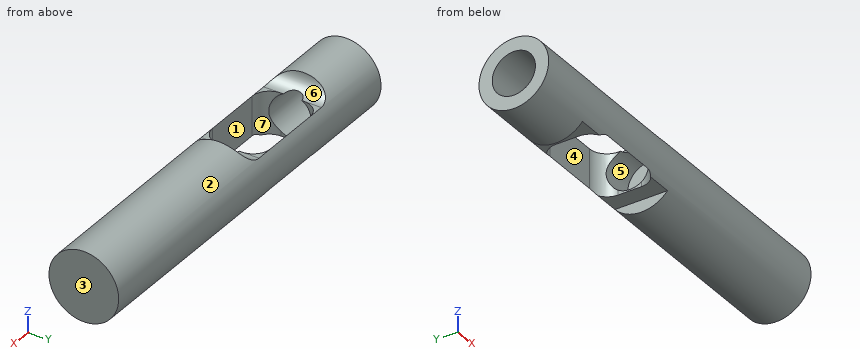
```python
from build123d import *

# Parameters (mm, degrees)
F0_W     = 115.125928
F0_H     = 10.15817
F2_W     = 37.343366
F2_H     = 12.383293
F3_DEPTH = 25
F4_R     = 6.295086
F5_DEPTH = 59.5
F7_DEPTH = 25


with BuildPart() as f1:
    # F0 (on Front) → F1 (revolve)
    with BuildSketch(Plane.XZ):
        with Locations((-1.547912, 5.079085)):
            Rectangle(F0_W, F0_H)
    revolve(axis=Axis((-1.547912, 0, 0), (-1, 0, 0)))

    # F2 (on Front) → F3 (cut, symmetric)
    with BuildSketch(Plane.XZ):
        with BuildLine():
            Line((-3.192568, 19.639129), (-40.535934, 19.639129))
            Line((-40.535934, 19.639129), (-40.535934, 10.707924))
            ThreePointArc((-40.535934, 10.707924), (-39.071468, 7.17239), (-35.535934, 5.707924))
            Line((-35.535934, 5.707924), (-8.192568, 5.707924))
            ThreePointArc((-8.192568, 5.707924), (-4.657034, 7.17239), (-3.192568, 10.707924))
            Line((-3.192568, 10.707924), (-3.192568, 19.639129))
        make_face()
        with Locations((-21.864251, -12.867015)):
            Rectangle(F2_W, F2_H)
    extrude(amount=F3_DEPTH, both=True, mode=Mode.SUBTRACT)

    # F4 (on face) → F5 (cut)
    with BuildSketch(Plane(origin=(-59.110876, 0, 0), x_dir=(0, -1, 0), z_dir=(-1, 0, 0))):
        Circle(F4_R)
    extrude(amount=-F5_DEPTH, mode=Mode.SUBTRACT)

    # F6 (on Top) → F7 (cut, symmetric)
    with BuildSketch(Plane.XY):
        with BuildLine():
            Line((-13.192568, 8.402858), (-30.535934, 8.402858))
            ThreePointArc((-30.535934, 8.402858), (-34.071468, 6.938392), (-35.535934, 3.402858))
            Line((-35.535934, 3.402858), (-35.535934, -3.402858))
            ThreePointArc((-35.535934, -3.402858), (-34.071468, -6.938392), (-30.535934, -8.402858))
            Line((-30.535934, -8.402858), (-13.192568, -8.402858))
            ThreePointArc((-13.192568, -8.402858), (-9.657034, -6.938392), (-8.192568, -3.402858))
            Line((-8.192568, -3.402858), (-8.192568, 3.402858))
            ThreePointArc((-8.192568, 3.402858), (-9.657034, 6.938392), (-13.192568, 8.402858))
        make_face()
    extrude(amount=F7_DEPTH, both=True, mode=Mode.SUBTRACT)


solid = f1.part
```
Geometry: final body of the model. Coordinates: model frame, mm. Face numbers are marked on the shaded views. A direction names the side the tool comes from. Coordinates: 2 decimals unless noted, no trailing zeros. Order: outer loops, then holes, each group sorted by start corner. A loop starts at its lowest first (then second) coordinate and runs counter-clockwise, first axis right, second up.
Item 1: Access query for the marked faces 5, 6 and 7. Directions: +Z, -Z, +X, -X, +Y, -Y. A direction counts if a zero-diameter tool reaches every point of the face in a straight line with its end or side. Return the directions, or none.
Answer:
face 5: -X
face 6: +Z, +Y, -Y
face 7: +Z, -Z
Item 2: Section query A-A (y = 0). Output: boundary loops of the cut face in (x, z), then the cut area to 3 significant figures.
Answer:
outline: (-59.11, -10.16) - (-40.54, -10.16) - (-40.54, -6.68) - (-35.54, -6.68) - (-35.54, -6.3) - (-59.11, -6.3) - close; (-59.11, 6.3) - (-37.89, 6.3) arc R5 cw to (-40.51, 10.16) - (-59.11, 10.16) - close; (-8.19, -6.68) - (-3.19, -6.68) - (-3.19, -10.16) - (56.02, -10.16) - (56.02, 10.16) - (-3.22, 10.16) arc R5 cw to (-5.84, 6.3) - (0.39, 6.3) - (0.39, -6.3) - (-8.19, -6.3) - close
area: 1,310 mm2
Item 3: Section query B-B (z = 4.25). Output: boundary loops of the cut face in (x, y).
Answer:
outline: (-59.11, -9.23) - (56.02, -9.23) - (56.02, 9.23) - (-59.11, 9.23) - (-59.11, 4.64) - (-35.38, 4.64) arc R5 cw to (-30.54, 8.4) - (-13.19, 8.4) arc R5 cw to (-8.35, 4.64) - (0.39, 4.64) - (0.39, -4.64) - (-8.35, -4.64) arc R5 cw to (-13.19, -8.4) - (-30.54, -8.4) arc R5 cw to (-35.38, -4.64) - (-59.11, -4.64) - close
Item 4: Contact query for flat-ended pins moving along their axis: P1, Ø8, axis at x = -8.5, y = 2, coming from the -Z side; P2, Ø5, axis at x = -41, z = 7, coming from the +Y side; P3, Ø5.5, axis at x = -10, y = -7, coming from the +Z side; P4, Ø2.5, axis at x = -32, y = 5, coming from the +Z side (1 decimal). Output: stop coordinate, or through.
Answer:
P1: stops at z = -6.68
P2: stops at y = 9.11
P3: stops at z = 5.8
P4: passes through
Item 5: Material intervals for line 1 along Z through (x, y) = (-3, 0); line 2 along X through (y, z) = (1, -0.5), sorted ascending.
Answer:
line 1: z = -10.16 to -6.3, 6.3 to 10.16
line 2: x = 0.39 to 56.02
Item 6: Section query C-C (y = 4.5). Output: boundary loops of the cut face in (x, z), then the cut area to 3 significant figures.
Answer:
outline: (-59.11, -9.11) - (-40.54, -9.11) - (-40.54, -6.68) - (-35.41, -6.68) - (-35.41, -4.4) - (-59.11, -4.4) - close; (-59.11, 4.4) - (-35.41, 4.4) - (-35.41, 5.71) - (-35.54, 5.71) arc R5 cw to (-40.27, 9.11) - (-59.11, 9.11) - close; (-8.31, -6.68) - (-3.19, -6.68) - (-3.19, -9.11) - (56.02, -9.11) - (56.02, 9.11) - (-3.46, 9.11) arc R5 cw to (-8.19, 5.71) - (-8.31, 5.71) - (-8.31, 4.4) - (0.39, 4.4) - (0.39, -4.4) - (-8.31, -4.4) - close
area: 1,270 mm2
Item 7: Section query D-D (x = -7). Output: boundary loops of the cut face in (y, z), then the cut area to 3 significant figures.
Answer:
outline: (-8.3, 5.85) arc R10.16 ccw to (-7.66, -6.68) - (7.66, -6.68) arc R10.16 ccw to (8.3, 5.85) - (2.32, 5.85) arc R6.3 cw (long way) to (-2.32, 5.85) - close
area: 114 mm2
Item 8: Draft query along X for the marked faces 1, 2, 3 and 4. Return one class per face: released by +X, released by -X, zero draft, split by the parting line, or undercut.
Answer:
face 1: undercut
face 2: zero draft
face 3: released by +X
face 4: undercut
